Design review of the part shown in the three views and the two pictorial views. Dimensions are in mm from the part's minimum x, y and z. A direction names the side the tool comes from. Round coordinates to 2 decimals unless told otherwise and drop trailing zeros. Write each loop counter-clockwise with the first axis right and the second up, starting at its lowest first coordinate (ties: lowest second). Pieces come first, ordered by that corner, then holes. Notation, with made-up numbers: (-38.5, 7.5) -> (-10.5, 7.5) arc R27 ccw to (-10.5, 46.5) -> close; hole circle Ø7 at (54, 19). An arc over 180 degrees is marked (long way). Answer as a JSON object with one key per item and string values. Group by question number.
1) Mouldability with a two-part tool opening along Y and no side actions: class the marked faces 1, 2 and 3 as pulls with the +Y half, pulls with the -Y half, needs draft (parallel to the pull), parting line crosses it, or undercut.
2) Insertion check: pin 1 Ø4 at (x, y) = (6, 7) entering from +Z; pin 2 Ø3 at (x, z) = (4, 2.5) entering from -Y; pin 3 Ø0.5 at (y, z) = (8, 10) entering from +X. Each pin has a flat end and moves straight along its axis. Give the tip position at first contact, or say it passes through.
3) We need section A-A, the plane x = 4.5. Write out the cut boundary in (y, z), then the cut area to 3 significant figures.
4) Machinability: for the marked faces 4, 5 and 6, which of the approach directions +Z, -Z, +X, -X, +Y, -Y give a long, thin tool a straight path to every point of the face, cutting with its end or side? Answer none if there is none.
5) To check wall thickness, follow probe 1 along Y at (x, z) = (3.5, 9.75); probe 2 along Z at (x, y) = (1.25, 11.5); probe 3 along X at (y, z) = (11, 2.25). State the ranges of each line that lie inside material, in increasing order. Write a range as [from, to].
6) We need section B-B, the plane y = 10. Write out the cut boundary in (x, z), then the cut area to 3 significant figures.
7) We need section C-C, the plane z = 5. Write out the cut boundary in (x, y), then the cut area to 3 significant figures.
8) We need section D-D, the plane z = 6.75. Write out the cut boundary in (x, y), then the cut area to 3 significant figures.
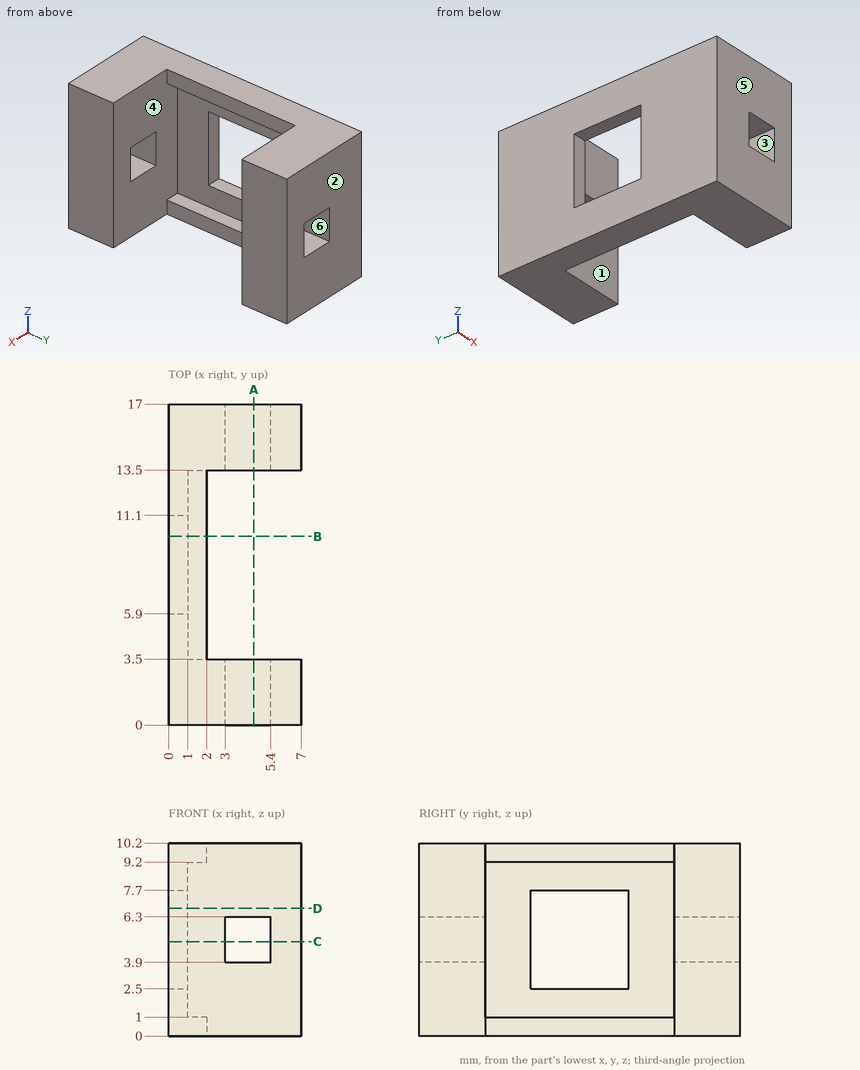
Here are the results:
{
 "1": {"face 1": "undercut", "face 2": "pulls with the +Y half", "face 3": "needs draft"},
 "2": {"pin 1": "passes through", "pin 2": "stops at y = 0", "pin 3": "stops at x = 2"},
 "3": {"outline": "(0, 0) -> (3.5, 0) -> (3.5, 3.9) -> (0, 3.9) -> close; (0, 6.3) -> (3.5, 6.3) -> (3.5, 10.2) -> (0, 10.2) -> close; (13.5, 0) -> (17, 0) -> (17, 3.9) -> (13.5, 3.9) -> close; (13.5, 6.3) -> (17, 6.3) -> (17, 10.2) -> (13.5, 10.2) -> close", "area": "54.6 mm^2"},
 "4": {"face 4": "+X", "face 5": "+Z, -Z, +X, -X, -Y", "face 6": "+Y, -Y"},
 "5": {"probe 1": "y = [0, 3.5], [13.5, 17]", "probe 2": "z = [0, 1], [9.2, 10.2]", "probe 3": "x = [0, 1]"},
 "6": {"outline": "(0, 0) -> (2, 0) -> (2, 1) -> (1, 1) -> (1, 2.5) -> (0, 2.5) -> close; (0, 7.7) -> (1, 7.7) -> (1, 9.2) -> (2, 9.2) -> (2, 10.2) -> (0, 10.2) -> close", "area": "7.00 mm^2"},
 "7": {"outline": "(0, 0) -> (3, 0) -> (3, 3.5) -> (1, 3.5) -> (1, 5.9) -> (0, 5.9) -> close; (0, 11.1) -> (1, 11.1) -> (1, 13.5) -> (3, 13.5) -> (3, 17) -> (0, 17) -> close; (5.4, 0) -> (7, 0) -> (7, 3.5) -> (5.4, 3.5) -> close; (5.4, 13.5) -> (7, 13.5) -> (7, 17) -> (5.4, 17) -> close", "area": "37.0 mm^2"},
 "8": {"outline": "(0, 0) -> (7, 0) -> (7, 3.5) -> (1, 3.5) -> (1, 5.9) -> (0, 5.9) -> close; (0, 11.1) -> (1, 11.1) -> (1, 13.5) -> (7, 13.5) -> (7, 17) -> (0, 17) -> close", "area": "53.8 mm^2"}
}
